```python
from build123d import *

# Parameters (mm, degrees)
SKETCH_1_W          = 257
SKETCH_1_H          = 150
SKETCH_1_R          = 1.65
EXTRUDE_1_DEPTH     = 3
CUT_EXTRUDE_1_DEPTH = 298.58696208
FILLET_1_R          = 3
FILLET_2_R          = 5


with BuildPart() as part:
    # 草图1 → 凸台-拉伸1 (new body)
    with BuildSketch(Plane(origin=(0, 0, 0), x_dir=(1, 0, 0), z_dir=(0, 1, 0))):
        with Locations((128.5, 75)):
            Rectangle(SKETCH_1_W, SKETCH_1_H)
        with Locations(Location((4.7, 45, 0), (0, 0, 270))):
            Circle(SKETCH_1_R, mode=Mode.SUBTRACT)
        with Locations(Location((4.7, 105, 0), (0, 0, 270))):
            Circle(SKETCH_1_R, mode=Mode.SUBTRACT)
        with Locations(Location((45.3, 45, 0), (0, 0, 270))):
            Circle(SKETCH_1_R, mode=Mode.SUBTRACT)
        with Locations(Location((45.3, 105, 0), (0, 0, 270))):
            Circle(SKETCH_1_R, mode=Mode.SUBTRACT)
        with Locations(Location((252.3, 105, 0), (0, 0, 90))):
            Circle(SKETCH_1_R, mode=Mode.SUBTRACT)
        with Locations(Location((211.7, 105, 0), (0, 0, 90))):
            Circle(SKETCH_1_R, mode=Mode.SUBTRACT)
        with Locations(Location((252.3, 45, 0), (0, 0, 90))):
            Circle(SKETCH_1_R, mode=Mode.SUBTRACT)
        with Locations(Location((211.7, 45, 0), (0, 0, 90))):
            Circle(SKETCH_1_R, mode=Mode.SUBTRACT)
        with BuildLine():
            Line((6.4, 137), (6.4, 125))
            ThreePointArc((6.4, 125), (4.7, 123.3), (3, 125))
            Line((3, 125), (3, 137))
            ThreePointArc((3, 137), (4.7, 138.7), (6.4, 137))
        make_face(mode=Mode.SUBTRACT)
        with BuildLine():
            Line((43.6, 137), (43.6, 125))
            ThreePointArc((43.6, 125), (45.3, 123.3), (47, 125))
            Line((47, 125), (47, 137))
            ThreePointArc((47, 137), (45.3, 138.7), (43.6, 137))
        make_face(mode=Mode.SUBTRACT)
        with BuildLine():
            Line((43.6, 13), (43.6, 25))
            ThreePointArc((43.6, 25), (45.3, 26.7), (47, 25))
            Line((47, 25), (47, 13))
            ThreePointArc((47, 13), (45.3, 11.3), (43.6, 13))
        make_face(mode=Mode.SUBTRACT)
        with BuildLine():
            Line((6.4, 13), (6.4, 25))
            ThreePointArc((6.4, 25), (4.7, 26.7), (3, 25))
            Line((3, 25), (3, 13))
            ThreePointArc((3, 13), (4.7, 11.3), (6.4, 13))
        make_face(mode=Mode.SUBTRACT)
        with BuildLine():
            Line((213.4, 13), (213.4, 25))
            ThreePointArc((213.4, 25), (211.7, 26.7), (210, 25))
            Line((210, 25), (210, 13))
            ThreePointArc((210, 13), (211.7, 11.3), (213.4, 13))
        make_face(mode=Mode.SUBTRACT)
        with BuildLine():
            Line((250.6, 13), (250.6, 25))
            ThreePointArc((250.6, 25), (252.3, 26.7), (254, 25))
            Line((254, 25), (254, 13))
            ThreePointArc((254, 13), (252.3, 11.3), (250.6, 13))
        make_face(mode=Mode.SUBTRACT)
        with BuildLine():
            Line((250.6, 137), (250.6, 125))
            ThreePointArc((250.6, 125), (252.3, 123.3), (254, 125))
            Line((254, 125), (254, 137))
            ThreePointArc((254, 137), (252.3, 138.7), (250.6, 137))
        make_face(mode=Mode.SUBTRACT)
        with BuildLine():
            Line((213.4, 137), (213.4, 125))
            ThreePointArc((213.4, 125), (211.7, 123.3), (210, 125))
            Line((210, 125), (210, 137))
            ThreePointArc((210, 137), (211.7, 138.7), (213.4, 137))
        make_face(mode=Mode.SUBTRACT)
    extrude(amount=EXTRUDE_1_DEPTH)

    # 草图2 → 切除-拉伸1 (cut, through all)
    with BuildSketch(Plane(origin=(0, 3, 0), x_dir=(1, 0, 0), z_dir=(0, 1, 0))):
        Polygon((57, 140), (123.5, 140), (57, 92.306014173), align=None)
        Polygon((57, 80), (123.5, 127.693985827), (123.5, 80), align=None)
        Polygon((133.5, 80), (200, 80), (133.5, 127.693985827), align=None)
        Polygon((200, 92.306014173), (200, 140), (133.5, 140), align=None)
        Polygon((200, 10), (133.5, 10), (200, 57.693985827), align=None)
        Polygon((200, 70), (133.5, 22.306014173), (133.5, 70), align=None)
        Polygon((123.5, 70), (57, 70), (123.5, 22.306014173), align=None)
        Polygon((57, 57.693985827), (57, 10), (123.5, 10), align=None)
    extrude(amount=-CUT_EXTRUDE_1_DEPTH, mode=Mode.SUBTRACT)

    # 圆角1
    fillet_1_edges = [part.edges().sort_by_distance(p)[0] for p in [
        (200, 1.5, -57.693985827),
        (200, 1.5, -10),
        (133.5, 1.5, -10),
        (200, 1.5, -92.306014173),
        (133.5, 1.5, -140),
        (200, 1.5, -140),
        (133.5, 1.5, -80),
        (133.5, 1.5, -127.693985827),
        (200, 1.5, -80),
        (123.5, 1.5, -80),
        (57, 1.5, -80),
        (123.5, 1.5, -127.693985827),
        (57, 1.5, -57.693985827),
        (123.5, 1.5, -10),
        (57, 1.5, -10),
        (123.5, 1.5, -70),
        (123.5, 1.5, -22.306014173),
        (57, 1.5, -70),
        (133.5, 1.5, -70),
        (200, 1.5, -70),
        (133.5, 1.5, -22.306014173),
        (57, 1.5, -92.306014173),
        (57, 1.5, -140),
        (123.5, 1.5, -140),
    ]]
    fillet(fillet_1_edges, radius=FILLET_1_R)

    # 圆角2
    fillet_2_edges = [part.edges().sort_by_distance(p)[0] for p in [
        (0, 1.5, -150),
        (257, 1.5, -150),
        (257, 1.5, 0),
        (0, 1.5, 0),
    ]]
    fillet(fillet_2_edges, radius=FILLET_2_R)


solid = part.part
```
The listing builds one solid part. Answer for the finished solid, in the listing's coordinates (mm). A direction names the side the tool comes from. Give positions to 0.01 mm unless a question says otherwise; leave off trailing zeros. Loops run counter-clockwise (first coordinate to the right, second up) from the corner with the lowest first, then second, coordinate; pieces in that order, holes last. Notation, with made-up numbers: (23.25, 19.5) - (39.25, 19.5) arc R20 ccw to (39.25, 46.5) - close; hole circle Ø4 at (12, -4). An arc over 180 degrees is marked (long way). Answer as CSV lines item,"result". Start each with the question number.
Item 1: Find the intervals of material crossed by line 1 (Z direction, x = 136, y = 0.9); line 2 (Z direction, x = 211.7, y = 0.75); line 3 (X direction, y = 0.7, z = -65.5), in increasing order. Write a range as from..to.
Item 2: A cutting plane is placed at C-C on y = 0.5. Count the separate pieces of the cut face and the enclosed holes in it, then the cut area to 3 significant figures.
Item 3: A cutting plane is placed at B-B on x = 146.5. Determine the outline of the cut face in (y, z), then the cut area to 3 significant figures.
Item 4: A cutting plane is placed at A-A on z = -116.5. Determine the outline of the cut face in (x, y).
Item 5: The mould has two halves that part along X. Classify faces 3 (the face through (1, 2, -148)), 4 (the face through (91.3, 1.5, -104.6)), 5 (the face through (127, 0, -76)): +X half, -X half, draft (parallel to the pull), parting line (faces both ways), or undercut.
Item 6: For faces 1 (the face through (165.7, 1.5, -104.6)), 2 (the face through (255, 2, -1)), determine the directions among +Z, -Z, +X, -X, +Y, -Y from which every point of the face is accessible in a straight line to the end or side of a thin tool.
Found:
1,line 1,"z = -150..-124.81, -80.04..-69.96, -25.19..0"
1,line 2,"z = -150..-138.7, -123.3..-106.65, -103.35..-46.65, -43.35..-26.7, -11.3..0"
1,line 3,"x = 0..63.73, 123.5..133.5, 193.27..257"
2,separate pieces,"1"
2,enclosed holes,"24"
2,area,"25,600 mm^2"
3,outline,"(0, -150) - (3, -150) - (3, -140) - (0, -140) - close; (0, -130.68) - (3, -130.68) - (3, -118.37) - (0, -118.37) - close; (0, -80) - (3, -80) - (3, -70) - (0, -70) - close; (0, -31.63) - (3, -31.63) - (3, -19.32) - (0, -19.32) - close; (0, -10) - (3, -10) - (3, 0) - (0, 0) - close"
3,area,"164 mm^2"
4,outline,"(0, 0) - (57, 0) - (57, 3) - (0, 3) - close; (90.73, 0) - (107.89, 0) - (107.89, 3) - (90.73, 3) - close; (123.5, 0) - (133.5, 0) - (133.5, 3) - (123.5, 3) - close; (149.11, 0) - (166.27, 0) - (166.27, 3) - (149.11, 3) - close; (200, 0) - (257, 0) - (257, 3) - (200, 3) - close"
5,face 3,"-X half"
5,face 4,"undercut"
5,face 5,"draft"
6,face 1,"+Y, -Y"
6,face 2,"+Z, +X, +Y, -Y"
